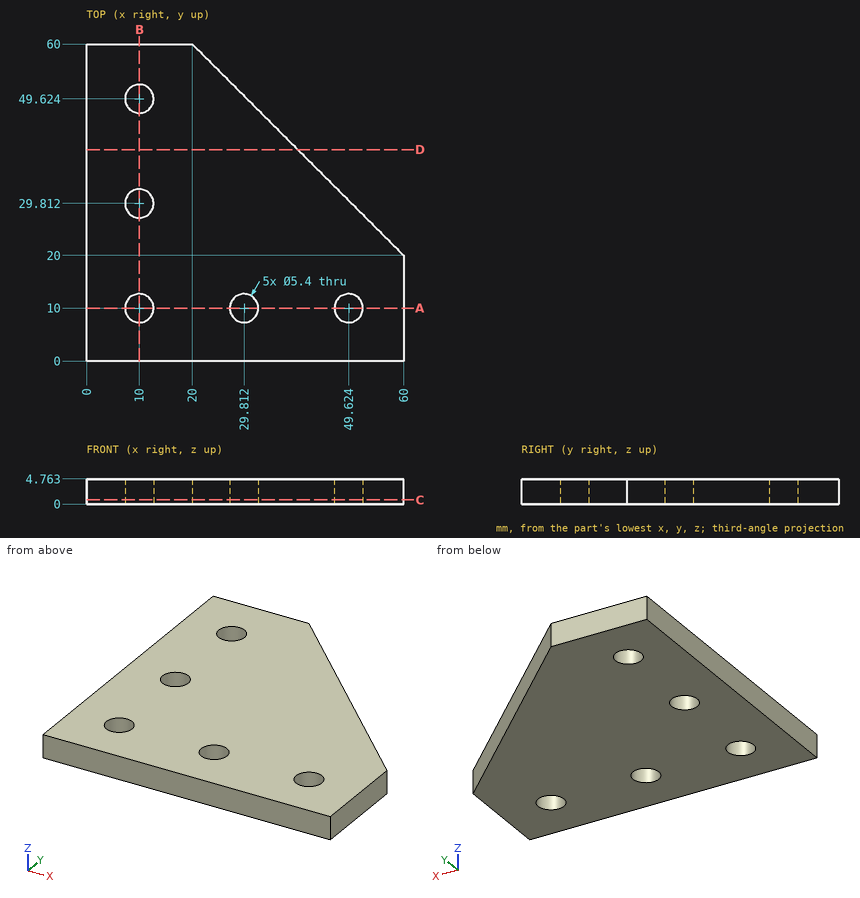
Check sheet for the drawn part. Datum: minimum x, y, z corner. Units: mm. Give positions to 0.01 mm unless a question says otherwise; leave off trailing zeros. Write each loop counter-clockwise with the first axis right and the second up, starting at its lowest first coordinate (ties: lowest second). Pieces come first, ordered by that corner, then holes. Notation, with made-up numbers: (5.25, 86) - (10.25, 86) arc R31 ccw to (10.25, 117) - close; hole circle Ø3 at (43, 40.5). An arc over 180 degrees is marked (long way). Put each result on its own line as item: value.
1. Sectioned sample at D-D, the plane y = 40. Enter the section's corners in (x, z).
Ans:
outline: (0, 0) - (40, 0) - (40, 4.76) - (0, 4.76) - close
2. Thickness scan on line 1 (Y direction, x = 10, z = 3.6) (1 decimal); line 2 (Y direction, x = 12, z = 1.8) (1 decimal). Record the ranges inside material, lowest first.
Ans:
line 1: y = 0 to 7.3, 12.7 to 27.1, 32.5 to 46.9, 52.3 to 60
line 2: y = 0 to 8.2, 11.8 to 28, 31.6 to 47.8, 51.4 to 60
3. Sectioned sample at C-C, the plane z = 0.8. Enter the section's corners in (x, y) (1 decimal).
Ans:
outline: (0, 0) - (60, 0) - (60, 20) - (20, 60) - (0, 60) - close; hole circle Ø5.4 at (10, 10); hole circle Ø5.4 at (10, 29.8); hole circle Ø5.4 at (10, 49.6); hole circle Ø5.4 at (29.8, 10); hole circle Ø5.4 at (49.6, 10)
4. Sectioned sample at A-A, the plane y = 10. Enter the section's corners in (x, z) (1 decimal).
Ans:
outline: (0, 0) - (7.3, 0) - (7.3, 4.8) - (0, 4.8) - close; (12.7, 0) - (27.1, 0) - (27.1, 4.8) - (12.7, 4.8) - close; (32.5, 0) - (46.9, 0) - (46.9, 4.8) - (32.5, 4.8) - close; (52.3, 0) - (60, 0) - (60, 4.8) - (52.3, 4.8) - close
